Check sheet for the modelled part. Datum: model origin and axes. Units: mm. Face numbers are marked on the shaded views. A direction names the side the tool comes from. Round coordinates to 2 decimals unless told otherwise and drop trailing zeros. Loops run counter-clockwise (first coordinate to the right, second up) from the corner with the lowest first, then second, coordinate; pieces in that order, holes last. Notation, with made-up numbers: (66.5, 41.25) -> (106.5, 41.25) arc R25 ccw to (106.5, 54.25) -> close; hole circle Ø2 at (59, 51.25). An arc over 180 degrees is marked (long way). One line per question, with ' | ' between items.
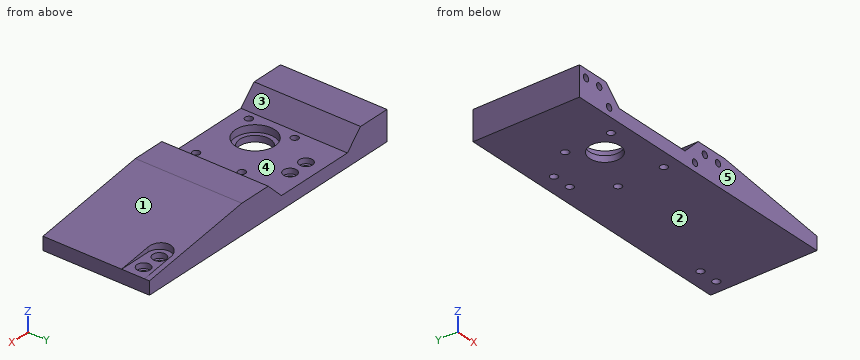
```python
from build123d import *

# Parameters (mm, degrees)
BOSS_EXTRUDE1_DEPTH                                 = 65
F_4_0MM_DOWEL_HOLE1_D                               = 4
F_4_0MM_DOWEL_HOLE1_DEPTH                           = 7.1
F_4_0MM_DOWEL_HOLE1_TIP                             = 1.201721238
CUT_EXTRUDE1_START                                  = 8
CUT_EXTRUDE1_DEPTH                                  = 8
CBORE_FOR_M4_HEX_SOCKET_HEAD_CAP_SCREW1_D           = 4.5
CBORE_FOR_M4_HEX_SOCKET_HEAD_CAP_SCREW1_DEPTH       = 8
CBORE_FOR_M4_HEX_SOCKET_HEAD_CAP_SCREW1_CBORE_D     = 8
CBORE_FOR_M4_HEX_SOCKET_HEAD_CAP_SCREW1_CBORE_DEPTH = 3.2
SKETCH8_R                                           = 12
CUT_EXTRUDE2_DEPTH                                  = 4.3
CUT_EXTRUDE3_REACH                                  = 5.7
SKETCH9_R                                           = 9.3
M4_CLEARANCE_HOLE1_D                                = 4.5
M4_CLEARANCE_HOLE1_DEPTH                            = 8


with BuildPart() as part:
    # Sketch2 → Boss-Extrude1 (new body)
    with BuildSketch(Plane(origin=(0, 0, 0), x_dir=(1, 0, 0), z_dir=(0, 1, 0))):
        Polygon((180, 0), (0, 0), (0, -18), (20, -18), (30, -8), (80, -8), (90, -18), (110, -18), (180, -8), align=None)
    extrude(amount=BOSS_EXTRUDE1_DEPTH)

    # Ø4.0mm Dowel Hole1
    with Locations(Plane(origin=(0, 0, 0), x_dir=(-1, 0, 0), z_dir=(0, -1, 0))):
        with Locations((-5, -13), (-15, -13), (-95, -13), (-105, -13), (-22.5, -5), (-87.5, -5)):
            Hole(F_4_0MM_DOWEL_HOLE1_D / 2, depth=F_4_0MM_DOWEL_HOLE1_DEPTH)
            with Locations((0, 0, -(F_4_0MM_DOWEL_HOLE1_DEPTH + F_4_0MM_DOWEL_HOLE1_TIP / 2))):  # 118° drill point
                Cone(0, F_4_0MM_DOWEL_HOLE1_D / 2, F_4_0MM_DOWEL_HOLE1_TIP, mode=Mode.SUBTRACT)

    # Sketch5 → Cut-Extrude1 (cut)
    with BuildSketch(Plane.XY.offset(CUT_EXTRUDE1_START)):
        with BuildLine():
            Line((180, 48), (160, 48))
            ThreePointArc((160, 48), (153, 55), (160, 62))
            Line((160, 62), (180, 62))
            ThreePointArc((180, 62), (187, 55), (180, 48))
        make_face()
    extrude(amount=CUT_EXTRUDE1_DEPTH, mode=Mode.SUBTRACT)

    # CBORE for M4 Hex Socket Head Cap Screw1
    with Locations(Plane.XY.offset(8)):
        with Locations((160, 55), (172, 55), (49, 55), (61, 55)):
            CounterBoreHole(CBORE_FOR_M4_HEX_SOCKET_HEAD_CAP_SCREW1_D / 2, CBORE_FOR_M4_HEX_SOCKET_HEAD_CAP_SCREW1_CBORE_D / 2, CBORE_FOR_M4_HEX_SOCKET_HEAD_CAP_SCREW1_CBORE_DEPTH, depth=CBORE_FOR_M4_HEX_SOCKET_HEAD_CAP_SCREW1_DEPTH)

    # Sketch8 → Cut-Extrude2 (cut)
    with BuildSketch(Plane.XY.offset(8)):
        with Locations((46.8, 22.15)):
            Circle(SKETCH8_R)
    extrude(amount=-CUT_EXTRUDE2_DEPTH, mode=Mode.SUBTRACT)

    # Sketch9 → Cut-Extrude3 (cut, up to next)
    with BuildSketch(Plane.XY.offset(3.7), mode=Mode.PRIVATE) as cut_extrude3_sk1:
        with Locations((46.8, 22.15)):
            Circle(SKETCH9_R)
    cut_extrude3_tool1 = extrude(cut_extrude3_sk1.sketch, amount=-CUT_EXTRUDE3_REACH, mode=Mode.PRIVATE) & part.part
    add(cut_extrude3_tool1.solids().sort_by_distance((46.8, 22.15, 3.7))[0], mode=Mode.SUBTRACT)

    # M4 Clearance Hole1
    with Locations(Plane.XY.offset(8)):
        with Locations((35, 36.853925583), (75, 36.853925583), (75, 8.853925583), (35, 8.853925583)):
            Hole(M4_CLEARANCE_HOLE1_D / 2, depth=M4_CLEARANCE_HOLE1_DEPTH)


solid = part.part
```
(1) Sectioned sample at B-B, the plane y = 15.5. Record the cut outline in (x, z), and give its area (3 significant figures).
Answer:
outline: (0, 0) -> (40.3, 0) -> (40.3, 3.7) -> (36.81, 3.7) -> (36.81, 8) -> (30, 8) -> (20, 18) -> (0, 18) -> close; (53.3, 0) -> (180, 0) -> (180, 8) -> (110, 18) -> (90, 18) -> (80, 8) -> (56.79, 8) -> (56.79, 3.7) -> (53.3, 3.7) -> close | area: 2,160 mm2
(2) Sectioned sample at D-D, the plane x = 144. Record the cut outline in (y, z).
Answer:
outline: (0, 0) -> (65, 0) -> (65, 13.14) -> (0, 13.14) -> close
(3) Go/stop test with flat-tipped pins: pin 1 (2.5 mm diameter, centred on x = 5, z = 13, fed in from -Y); pin 2 (1 mm diameter, centred on x = 156.5, y = 50, fed in from -Z); pin 3 (6 mm diameter, centred on x = 49, y = 55, fed in from +Z); pin 4 (9 mm diameter, centred on x = 61.5, y = 55.5, fed in from +Z). Record where each tip stops, or that it passes through.
Answer:
pin 1: stops at y = 7.55 | pin 2: stops at z = 0 | pin 3: stops at z = 4.8 | pin 4: stops at z = 8
(4) Sectioned sample at C-C, the plane y = 55. Count the separate pieces of the cut face and the enclosed holes in it, and give its area (3 significant figures).
Answer:
separate pieces: 5 | enclosed holes: 0 | area: 2,050 mm2
(5) Sectioned sample at A-A, the plane x = 61. Record the cut outline in (y, z), and give its area (3 significant figures).
Answer:
outline: (0, 0) -> (52.75, 0) -> (52.75, 4.8) -> (51, 4.8) -> (51, 8) -> (0, 8) -> close; (57.25, 0) -> (65, 0) -> (65, 8) -> (59, 8) -> (59, 4.8) -> (57.25, 4.8) -> close | area: 473 mm2
(6) Scan lines: probe 1 along Y at (x, z) = (75, 3.5); probe 2 along Y at (x, z) = (61, 1.1); probe 3 along Z at (x, y) = (5, 3.5). Record each from-to range of solid material in increasing order.
Answer:
probe 1: y = 0 to 6.6, 11.1 to 34.6, 39.1 to 65 | probe 2: y = 0 to 52.75, 57.25 to 65 | probe 3: z = 0 to 11, 15 to 18
(7) Mould release check, pull along X, two halves, no side actions. Record for the marked faces 1, 2 and 3: +X half, -X half, draft (parallel to the pull), parting line (faces both ways), or undercut.
Answer:
face 1: +X half | face 2: draft | face 3: undercut
(8) Set-up check for the marked faces 4 and 5: record each of +Z, -Z, +X, -X, +Y, -Y from which the full face is reachable in a straight line by a thin tool's end or side.
Answer:
face 4: +Z, +Y, -Y | face 5: +Z, -Z, +X, -X, -Y
